from build123d import *

# Parameters (mm, degrees)
SKETCH1_W           = 20
SKETCH1_H           = 40
BOSS_EXTRUDE1_DEPTH = 6
CUT_EXTRUDE1_DEPTH  = 8
CUT_EXTRUDE2_DEPTH  = 2.86
CUT_EXTRUDE3_DEPTH  = 0.8
CUT_EXTRUDE4_DEPTH  = 45.870876969
SKETCH8_W           = 5
SKETCH8_H           = 8
BOSS_EXTRUDE2_DEPTH = 1
RIB2_REACH          = 44
SKETCH9_WALL_W      = 106.615528128
SKETCH9_WALL_H      = 5
SHELL1_START        = 1
SHELL1_DEPTH        = 4
SHELL1_2_DEPTH      = 0.34
SHELL1_START_2      = 4.14
SHELL1_3_DEPTH      = 0.86
SHELL1_START_3      = 8.5
SHELL1_4_DEPTH      = 3


with BuildPart() as part:
    # Sketch1 → Boss-Extrude1 (new body)
    with BuildSketch(Plane.XY):
        with Locations((10, 20)):
            Rectangle(SKETCH1_W, SKETCH1_H)
    extrude(amount=BOSS_EXTRUDE1_DEPTH)

    # Sketch2 → Cut-Extrude1 (cut)
    with BuildSketch(Plane(origin=(0, 40, 0), x_dir=(1, 0, 0), z_dir=(0, 1, 0))):
        Polygon((12.665, -2.34), (12.665, -3.14), (12.335, -3.14), (12.335, -6), (7.665, -6), (7.665, -3.14), (7.335, -3.14), (7.335, -2.34), (8.5, -2.34), (8.5, 0), (11.5, 0), (11.5, -2.34), align=None)
    extrude(amount=-CUT_EXTRUDE1_DEPTH, mode=Mode.SUBTRACT)

    # Sketch3 → Cut-Extrude2 (cut)
    with BuildSketch(Plane.XY.offset(6)):
        with BuildLine():
            Line((7.665, 32), (12.335, 32))
            ThreePointArc((12.335, 32), (10, 29.665), (7.665, 32))
        make_face()
    extrude(amount=-CUT_EXTRUDE2_DEPTH, mode=Mode.SUBTRACT)

    # Sketch5 → Cut-Extrude3 (cut)
    with BuildSketch(Plane.XY.offset(3.14)):
        with BuildLine():
            Line((7.335, 32), (12.665, 32))
            ThreePointArc((12.665, 32), (10, 29.335), (7.335, 32))
        make_face()
    extrude(amount=-CUT_EXTRUDE3_DEPTH, mode=Mode.SUBTRACT)

    # Sketch7 → Cut-Extrude4 (cut, through all)
    with BuildSketch(Plane.XY.offset(2.34)):
        with BuildLine():
            Line((9.77, 30.73), (9.77, 32))
            Line((9.77, 32), (10.23, 32))
            Line((10.23, 32), (10.23, 30.73))
            ThreePointArc((10.23, 30.73), (10, 30.5), (9.77, 30.73))
        make_face()
        with BuildLine():
            Line((8.5, 32), (8.96, 32))
            ThreePointArc((8.96, 32), (8.73, 31.77), (8.5, 32))
        make_face()
        with BuildLine():
            Line((11.04, 32), (11.5, 32))
            ThreePointArc((11.5, 32), (11.27, 31.77), (11.04, 32))
        make_face()
    extrude(amount=-CUT_EXTRUDE4_DEPTH, mode=Mode.SUBTRACT)

    # Sketch8 → Boss-Extrude2 (add)
    with BuildSketch(Plane.XZ):
        with Locations((10, -4)):
            Rectangle(SKETCH8_W, SKETCH8_H)
    boss_extrude2 = extrude(amount=-BOSS_EXTRUDE2_DEPTH)

    # Sketch9 wall → Rib2 (add, up to next)
    with BuildSketch(Plane(origin=(10, 10.5, -4), x_dir=(0, 0.921635375138, 0.388057000058), z_dir=(0, -0.388057000058, 0.921635375138)), mode=Mode.PRIVATE) as rib2_sk1:
        Rectangle(SKETCH9_WALL_W, SKETCH9_WALL_H)
    rib2_tool1 = extrude(rib2_sk1.sketch, amount=RIB2_REACH, mode=Mode.PRIVATE) - part.part
    rib2 = rib2_tool1.solids().sort_by_distance((10, 10.5, -4))[0]
    add(rib2)

    # Mirror1: Boss-Extrude2, Rib2 across plane
    add(boss_extrude2.mirror(Plane.XY.offset(3)))
    add(rib2.mirror(Plane.XY.offset(3)))

    # Shell1: read off the stored shape, not the designer's step
    # Shell1 outline → Shell1 (cut)
    with BuildSketch(Plane.XY.offset(SHELL1_START)):
        with BuildLine():
            Line((6.335, 32), (6.335, 39))
            Line((6.335, 39), (1, 39))
            Line((1, 39), (1, 0))
            Line((1, 0), (8.5, 0))
            Line((8.5, 0), (11.5, 0))
            Line((11.5, 0), (19, 0))
            Line((19, 0), (19, 39))
            Line((19, 39), (13.665, 39))
            Line((13.665, 39), (13.665, 32))
            ThreePointArc((13.665, 32), (10, 28.335), (6.335, 32))
        make_face()
    extrude(amount=SHELL1_DEPTH, mode=Mode.SUBTRACT)

    # Shell1 2 outline → Shell1 2 (cut)
    with BuildSketch(Plane.XY.offset(SHELL1_START)):
        with BuildLine():
            Line((7.5, 32), (7.5, 39))
            Line((7.5, 39), (6.335, 39))
            Line((6.335, 39), (6.335, 32))
            ThreePointArc((6.335, 32), (10, 28.335), (13.665, 32))
            Line((13.665, 32), (13.665, 39))
            Line((13.665, 39), (12.5, 39))
            Line((12.5, 39), (12.5, 32))
            ThreePointArc((12.5, 32), (12.12548232, 31.116229668), (11.23, 30.770650579))
            Line((11.23, 30.770650579), (11.23, 30.73))
            ThreePointArc((11.23, 30.73), (10, 29.5), (8.77, 30.73))
            Line((8.77, 30.73), (8.77, 30.770650579))
            ThreePointArc((8.77, 30.770650579), (7.87451768, 31.116229668), (7.5, 32))
        make_face()
    extrude(amount=SHELL1_2_DEPTH, mode=Mode.SUBTRACT)

    # Shell1 3 outline → Shell1 3 (cut)
    with BuildSketch(Plane.XY.offset(SHELL1_START_2)):
        with BuildLine():
            Line((6.665, 32), (6.665, 39))
            Line((6.665, 39), (6.335, 39))
            Line((6.335, 39), (6.335, 32))
            ThreePointArc((6.335, 32), (10, 28.335), (13.665, 32))
            Line((13.665, 32), (13.665, 39))
            Line((13.665, 39), (13.335, 39))
            Line((13.335, 39), (13.335, 32))
            ThreePointArc((13.335, 32), (10, 28.665), (6.665, 32))
        make_face()
    extrude(amount=SHELL1_3_DEPTH, mode=Mode.SUBTRACT)

    # Shell1 4 outline → Shell1 4 (cut)
    with BuildSketch(Plane.YZ.offset(SHELL1_START_3)):
        Polygon((0, 1), (0, -7), (0.798058984, -7), (19.798058984, 1), align=None)
        Polygon((0, 13), (0, 5), (19.798058984, 5), (0.798058984, 13), align=None)
    extrude(amount=SHELL1_4_DEPTH, mode=Mode.SUBTRACT)


solid = part.part
Verification items for the finished model (mm, model axes). A direction names the side the tool comes from. Give positions to 0.01 mm unless a question says otherwise; leave off trailing zeros. Order: outer loops, then holes, each group sorted by start corner. A loop starts at its lowest first (then second) coordinate and runs counter-clockwise, first axis right, second up. Notation, with made-up numbers: M 80,57.5 L 136,57.5 A22 ccw 136,66.5 Z; hole C 88.5,-29 d9. An arc over 180 degrees is marked long. Use one line per item in the form item = value. Start each with the question number.
Q1. Mould release check, pull along Z, two halves, no side actions. Record for faces 5 (the flat face through (8.5, 8, -2)), 6 (the flat face through (4, 40, 3)), 7 (the flat face through (9.9, 20.3, 0)): +Z half, -Z half, draft (parallel to the pull), parting line (faces both ways), or undercut.
Q2. Access from +Z, -Z, +X, -X, +Y, -Y to the whole of each face (thin tool, end or side, straight path). Record for faces 1 (the flat face through (9.4, 32, 1.2)), 2 (the flat face through (7.5, 7, -2)), 3 (the flat face through (7.335, 36.1, 2.7)), 4 (the flat face through (12, 20, 1)).
Q3. Section check A-A (y = 33). Count the separate pieces of the cut face and the enclosed holes in it, then the cut area to 3 significant figures.
Q4. Section check D-D (z = -4.5). Enter the section's corners in (x, y).
Q5. Section check C-C (x = 3). Enter the section's corners in (y, z).
Q6. Go/stop test with flat-tipped pins: pin 1 Ø4 at (y, z) = (13, -5) entering from -X; pin 2 Ø8 at (x, y) = (10.5, 36.5) entering from -Z; pin 3 Ø9 at (x, y) = (9.5, 14.5) entering from -Z. Record where each tip stops, or that it passes through.
Q7. Scan lines: line 1 along X through (y, z) = (38.5, 3.75) (3 decimals); line 2 along Z through (x, y) = (14, 37.5); line 3 along X through (y, z) = (2, 9.5). Record each from-to range of solid material in increasing order. Write a range as [from, to].
Q8. Section check B-B (y = 23.5). Enter the section's corners in (x, z), then the cut area to 3 significant figures.
Evaluation:
q1.face_5 = undercut
q1.face_6 = draft
q1.face_7 = -Z half
q2.face_1 = +Z, -Z, +Y
q2.face_2 = -Z, -X, +Y, -Y
q2.face_3 = +Y
q2.face_4 = -Y
q3.separate_pieces = 2
q3.enclosed_holes = 2
q3.area = 51.3 mm2
q4.outline = M 7.5,0 L 8.5,0 L 8.5,6.74 L 11.5,6.74 L 11.5,0 L 12.5,0 L 12.5,9.31 L 7.5,9.31 Z
q5.outline = M 0,0 L 40,0 L 40,6 L 0,6 L 0,5 L 39,5 L 39,1 L 0,1 Z
q6.pin_1 = 7.5
q6.pin_2 = 0
q6.pin_3 = -4.21
q7.line_1 = [0, 1], [6.335, 7.665], [12.335, 13.665], [19, 20]
q7.line_2 = [0, 1], [5, 6]
q7.line_3 = [7.5, 8.5], [11.5, 12.5]
q8.outline = M 0,0 L 20,0 L 20,6 L 0,6 Z; hole M 1,1 L 19,1 L 19,5 L 1,5 Z
q8.area = 48.0 mm2
